Verification items for the finished model (mm, model axes). A direction names the side the tool comes from. Round coordinates to 2 decimals unless told otherwise and drop trailing zeros. Write each loop counter-clockwise with the first axis right and the second up, starting at its lowest first coordinate (ties: lowest second). Pieces come first, ordered by that corner, then holes. Notation, with made-up numbers: M 70,3 L 76,3 A20 cw 76,7 Z; hole C 21,5 d2. An arc over 180 degrees is marked long. Write each question's results on one line, items separated by ' | '.
from build123d import *

# Parameters (mm, degrees)
SKETCH1_R           = 11
BOSS_EXTRUDE1_DEPTH = 9.525
SKETCH1_3_R         = 11
BOSS_EXTRUDE2_DEPTH = 2.52476
SKETCH2_R           = 4
CUT_EXTRUDE1_DEPTH  = 2.52476
SKETCH3_R           = 6.5
CUT_EXTRUDE2_DEPTH  = 10.525


with BuildPart() as part:
    # Sketch1 → Boss-Extrude1 (new body)
    with BuildSketch(Plane.XY):
        with BuildLine():
            ThreePointArc((12.610334109, 75.166477239), (0.013235783, 86.359993103), (-12.607166653, 75.192758621))
            Line((-12.607166653, 75.192758621), (-21.43218331, 2.605689655))
            ThreePointArc((-21.43218331, 2.605689655), (-1.305232229, -21.550509712), (21.59, 0))
            Line((21.59, 0), (12.610334109, 75.166477239))
        make_face()
        with Locations((0, 73.66)):
            Circle(SKETCH1_R, mode=Mode.SUBTRACT)
    extrude(amount=BOSS_EXTRUDE1_DEPTH)

    # Sketch1<3> → Boss-Extrude2 (add)
    with BuildSketch(Plane.XY):
        with Locations((0, 73.66)):
            Circle(SKETCH1_3_R)
    extrude(amount=BOSS_EXTRUDE2_DEPTH)

    # Sketch2 → Cut-Extrude1 (cut)
    with BuildSketch(Plane.XY.offset(2.52476)):
        with Locations((0, 73.66)):
            Circle(SKETCH2_R)
    extrude(amount=-CUT_EXTRUDE1_DEPTH, mode=Mode.SUBTRACT)

    # Sketch3 → Cut-Extrude2 (cut, through all)
    with BuildSketch(Plane.XY.offset(9.525)):
        Circle(SKETCH3_R)
    extrude(amount=-CUT_EXTRUDE2_DEPTH, mode=Mode.SUBTRACT)


solid = part.part
1) Access from +Z, -Z, +X, -X, +Y, -Y to the whole of each face (thin tool, end or side, straight path). Record for faces 1 (the flat face through (0, 33, 0)), 2 (the flat face through (5, 74, 2.525)).
Calculated:
face 1: -Z, +X, -X, +Y, -Y | face 2: +Z
2) Sectioned sample at D-D, the plane y = 73.66. Record the cut outline in (x, z) (3 decimals), and give its area (3 significant figures).
Calculated:
outline: M -12.794,0 L -4,0 L -4,2.525 L -11,2.525 L -11,9.525 L -12.794,9.525 Z; M 4,0 L 12.79,0 L 12.79,9.525 L 11,9.525 L 11,2.525 L 4,2.525 Z | area: 69.5 mm²
3) Sectioned sample at C-C, the plane z = 4.5. Record the cut outline in (x, y).
Calculated:
outline: M -21.43,2.61 A21.59 ccw long 21.59,0 L 12.61,75.17 A12.7 ccw -12.61,75.19 Z; hole C 0,73.66 d22; hole C 0,0 d13
4) Draft check along X on faces 3 (the cylindrical face through (-8.73, 66.97, 5.98)), 4 (the cylindrical face through (-0.521, 77.626, 1.28)), 5 (the flat face through (17.163, 37.057, 4.696)), 6 (the cylindrical face through (0.271, 86.357, 4.696)). Enter one of: pulls with the +X half, pulls with the -X half, needs draft (parallel to the pull), parting line crosses it, or undercut.
Calculated:
face 3: undercut | face 4: undercut | face 5: pulls with the +X half | face 6: parting line crosses it
5) Depth check by flat-ended pin: P1, Ø8, axis at x = 0, y = 0, coming from the -Z side; P2, Ø4, axis at y = 39.5, z = 2, coming from the +X side; P3, Ø5, axis at y = 23.5, z = 4, coming from the +X side. Enter the tip coordinate at first touch or a pass-through.
Calculated:
P1: passes through | P2: stops at x = 17.11 | P3: stops at x = 19.08
6) Sectioned sample at A-A, the plane x = 0. Record the cut outline in (y, z) (3 decimals).
Calculated:
outline: M -21.59,0 L -6.5,0 L -6.5,9.525 L -21.59,9.525 Z; M 6.5,0 L 69.66,0 L 69.66,2.525 L 62.66,2.525 L 62.66,9.525 L 6.5,9.525 Z; M 77.66,0 L 86.36,0 L 86.36,9.525 L 84.66,9.525 L 84.66,2.525 L 77.66,2.525 Z
7) Sectioned sample at B-B, the plane y = -3.5. Record the cut outline in (x, z) (3 decimals).
Calculated:
outline: M -21.304,0 L -5.477,0 L -5.477,9.525 L -21.304,9.525 Z; M 5.477,0 L 21.304,0 L 21.304,9.525 L 5.477,9.525 Z
8) Material ranges on line 1 (Y direction, x = 0, z = 4.5); line 2 (Y direction, x = 0, z = 1.4); line 3 (Y direction, x = 9.5, z = 3.5), recorded low to high. Write a range as [from, to].
Calculated:
line 1: y = [-21.59, -6.5], [6.5, 62.66], [84.66, 86.36] | line 2: y = [-21.59, -6.5], [6.5, 69.66], [77.66, 86.36] | line 3: y = [-19.39, 68.11], [79.21, 82.09]
